Input: part model. Units: mm. Frame: model coordinates. A direction names the side the tool comes from. Coordinates: 2 decimals unless noted, no trailing zeros. Loops run counter-clockwise (first coordinate to the right, second up) from the corner with the lowest first, then second, coordinate; pieces in that order, holes last.
Autodesk Inventor part; units mm, degrees
ref_plane "YZ Plane" through (0, 0, 0) normal (1, 0, 0) x (0, 1, 0)
ref_plane "XZ Plane" through (0, 0, 0) normal (0, 1, 0) x (-1, 0, 0)
ref_plane "XY Plane" through (0, 0, 0) normal (0, 0, 1) x (1, 0, 0)
sketch "Sketch1" plane through (0, 0, 0) normal (0, 0, 1) x (1, 0, 0)
  circle A0 centre (0, 0) radius 8.35 construction
  arc A1 (-8.8064, -7.1064) -> (-5.4064, -7.1064) centre (-7.1064, -7.1064) ccw
  circle A2 centre (7.1064, -7.1064) radius 1.7 construction
  line L0 (0, 12.3642) -> (0, -15.7353)
  line L1 (-7.1064, -8.8064) -> (7.1064, -8.8064) construction
  line L2 (0, 0) -> (7.1064, -7.1064) construction
  line L3 (11.8064, -3.7064) -> (11.8064, -11.7564)
  line L4 (11.8064, -11.7564) -> (-11.8064, -11.7564)
  line L5 (-11.8064, -11.7564) -> (-11.8064, -3.7064)
  circle A3 centre (-7.1064, -3.7064) radius 1.7 construction
  line L6 (-8.8064, -7.1064) -> (-8.8064, -3.7064)
  line L7 (-5.4064, -7.1064) -> (-5.4064, -3.7064)
  line L8 (-11.8064, -3.7064) -> (-8.8064, -3.7064)
  arc A4 (5.4064, -7.1064) -> (8.8064, -7.1064) centre (7.1064, -7.1064) ccw
  line L9 (8.8064, -7.1064) -> (8.8064, -3.7064)
  line L10 (5.4064, -7.1064) -> (5.4064, -3.7064)
  line L11 (-5.4064, -3.7064) -> (5.4064, -3.7064)
  line L12 (8.8064, -3.7064) -> (11.8064, -3.7064)
  dimension "d0" = 16.7
  dimension "d1" = 3.4
  dimension "d4" = 45
  dimension "d5" = 3
  dimension "d6" = 4.65
  dimension "d25" = 17.6129
extrude "Extrusion1" add sketch "Sketch1" along normal blind 60
sketch "Sketch2" plane through (5.4064, -7.1064, 0) normal (1, 0, 0) x (0, 0, -1)
  line L0 (0, -4.65) -> (0, 3.4)
  line L1 (0, 3.4) -> (-60, 3.4)
  line L2 (-60, -4.65) -> (-60, 3.4)
  line L3 (0, -4.65) -> (-60, -4.65)
  line L4 (0, 3.4) -> (-60, 3.4)
  circle A0 centre (-10, 3.4) radius 1.7
  point P0 (0, 7.1064)
  dimension "d9" = 10
  dimension "d10" = 3.4
extrude "Extrusion2" cut sketch "Sketch2" against normal up to surface (10.8128 mm away) contours A0 L1 | L1 A0
pattern_linear "Rectangular Pattern1" count 5 spacing 10 along (0, 0, 1) of "Extrusion2"
sketch "Sketch3" plane through (0, 0, 0) normal (0, 0, -1) x (-1, 0, 0)
  line L0 (11.8064, -3.7064) -> (11.8064, -11.7564)
  line L1 (8.8064, -3.7064) -> (11.8064, -3.7064)
  line L2 (8.8064, -7.1064) -> (8.8064, -3.7064)
  arc A0 (5.4064, -7.1064) -> (8.8064, -7.1064) centre (7.1064, -7.1064) ccw
  line L3 (5.4064, -3.7064) -> (5.4064, -7.1064)
  line L4 (-5.4064, -3.7064) -> (5.4064, -3.7064)
  line L5 (-5.4064, -7.1064) -> (-5.4064, -3.7064)
  arc A1 (-8.8064, -7.1064) -> (-5.4064, -7.1064) centre (-7.1064, -7.1064) ccw
  line L6 (-8.8064, -3.7064) -> (-8.8064, -7.1064)
  line L7 (-11.8064, -3.7064) -> (-8.8064, -3.7064)
  line L8 (-11.8064, -11.7564) -> (-11.8064, -3.7064)
  line L9 (11.8064, -11.7564) -> (-11.8064, -11.7564)
  arc A2 (0.375, -11.4658) -> (-0.375, -11.4658) centre (0, -9.7564) ccw
  line L10 (-0.375, -11.4658) -> (-0.375, -11.7564)
  line L11 (0.375, -11.4658) -> (0.375, -11.7564)
  point P0 (0, 0)
  dimension "d16" = 3.5
  dimension "d17" = 0.75
  dimension "d20" = 2
extrude "Extrusion3" cut sketch "Sketch3" against normal blind 30 contours L9 L10 A2 L11
sketch "Sketch4" plane through (-11.8064, -11.7564, 60) normal (0, -1, 0) x (1, 0, 0)
  line L0 (12.1814, -30) -> (12.1814, -60)
  line L1 (12.1814, -60) -> (23.6128, -60)
  line L2 (23.6128, -60) -> (23.6128, 0)
  line L3 (0, 0) -> (23.6128, 0)
  line L4 (0, -60) -> (0, 0)
  line L5 (0, -60) -> (11.4314, -60)
  line L6 (11.4314, -60) -> (11.4314, -30)
  line L7 (11.4314, -30) -> (12.1814, -30)
  line L8 (13.5064, -30) -> (10.1064, -30)
  line L9 (10.1064, -30) -> (10.1064, -33)
  line L10 (10.1064, -33) -> (13.5064, -33)
  line L11 (13.5064, -33) -> (13.5064, -30)
  line L12 (11.8064, 12) -> (11.8064, -72)
  point P0 (11.8064, -60)
  dimension "d21" = 3.4
  dimension "d22" = 3
extrude "Extrusion4" cut sketch "Sketch4" against normal blind 2 contours L8 L11 L10 L0 | L0 L10 L12 L7 | L12 L10 L6 L7 | L6 L10 L9 L8
sketch "Sketch5" plane through (0, 0, 0) normal (0, 0, -1) x (-1, 0, 0)
  line L0 (-11.8064, -11.7564) -> (-11.8064, -3.7064)
  circle A0 centre (-11.8064, -7.1064) radius 1.7
  line L1 (-0.375, -11.7564) -> (-11.8064, -11.7564)
  line L2 (-11.8064, -3.7064) -> (-8.8064, -3.7064)
  point P0 (0, 0)
  dimension "d26" = 3.4
  dimension "d28" = 3.4
extrude "Extrusion5" cut sketch "Sketch5" against normal up to surface (60 mm away)
sketch "Sketch6" plane through (11.8064, -11.7564, 60) normal (1, 0, 0) x (0, 0, -1)
  line L0 (60, 0) -> (0, 0)
  line L1 (60, 8.05) -> (0, 8.05)
  line L2 (40.7622, 0) -> (40.0122, 0)
  line L3 (40.0122, 0) -> (40.0122, 8.05)
  line L4 (40.0122, 8.05) -> (40.7622, 8.05)
  line L5 (40.7622, 8.05) -> (40.7622, 0)
  line L6 (60, 0) -> (0, 0) construction
  line L7 (40.3872, 0) -> (40.3872, 8.05) construction
  line L8 (60, 8.05) -> (60, 4.65)
  line L9 (60, 2.95) -> (0, 2.95)
  line L10 (60, 6.35) -> (58, 6.35)
  line L11 (58, 6.35) -> (58, 2.95)
  line L12 (58, 2.95) -> (60, 2.95)
  line L13 (60, 2.95) -> (60, 6.35)
  point P0 (60, 11.7564)
  dimension "d31" = 0.75
  dimension "d32" = 2
  dimension "d33" = 17.6129
extrude "Extrusion6" add sketch "Sketch6" against normal blind 1.7 contours L11 L10 L8 L13 L9
extrude "Extrusion7" cut sketch "Sketch6" against normal blind 1.7 contours L0 L3 L9 L5 | L9 L3 L1 L5
pattern_linear "Rectangular Pattern2" count 5 spacing 17.6128 along (0, 0, 1) of "Extrusion7"
sketch "Sketch7" plane through (-5.4064, -3.7064, 11.7) normal (0, 1, 0) x (1, 0, 0)
  point P0 (5.4064, 11.7)
equation "\"d0\" = marbleSize"
equation "\"d1\" = trackDiameter"
equation "\"d10\" = trackDiameter"
equation "\"d21\" = trackDiameter"
equation "\"d26\" = trackDiameter"
equation "\"d28\" = trackDiameter"
equation "\"d29\" = 0.5 * trackDiameter"
equation "\"d33\" = d25"
equation "\"d34\" = 0.5 * trackDiameter"
equation "\"d36\" = 0.5 * trackDiameter"
equation "\"d40\" = d25"
equation "\"marbleSize\" = 16.7"
equation "\"trackDiameter\" = 3.4"
equation "\"numGroove\" = 5"
properties part number "Track Builder"
Item 1: Section query D-D (z = 10). Output: boundary loops of the cut face in (x, y) (3 decimals), then the cut area to 3 significant figures.
Result:
outline: (-11.806, -11.756) - (-0.375, -11.756) - (-0.375, -11.466) arc R1.75 cw (long way) to (0.375, -11.466) - (0.375, -11.756) - (11.806, -11.756) - (11.806, -8.806) arc R1.7 cw to (11.806, -5.406) - (11.806, -3.706) - (8.806, -3.706) - (8.806, -7.106) arc R1.7 cw to (5.406, -7.106) - (5.406, -5.406) - (-5.406, -5.406) - (-5.406, -7.106) arc R1.7 cw to (-8.806, -7.106) - (-8.806, -3.706) - (-11.806, -3.706) - close
area: 125 mm2
Item 2: Section query A-A (z = 40). Output: boundary loops of the cut face in (x, y), then the cut area to 3 significant figures.
Result:
outline: (-11.81, -11.76) - (11.81, -11.76) - (11.81, -8.81) arc R1.7 cw to (11.81, -5.41) - (11.81, -3.71) - (8.81, -3.71) - (8.81, -7.11) arc R1.7 cw to (5.41, -7.11) - (5.41, -5.41) - (-5.41, -5.41) - (-5.41, -7.11) arc R1.7 cw to (-8.81, -7.11) - (-8.81, -3.71) - (-11.81, -3.71) - close
area: 135 mm2
Item 3: Line query: L1, parallel to X at y = -5, z = 12; L2, parallel to X at y = -8.5, z = 49.5; L3, parallel to X at y = -8.5, z = 19. Output: solid intervals per line, ascending.
Result:
L1: x = -11.81 to -8.81, -5.41 to 5.41, 8.81 to 11.81
L2: x = -11.81 to -8.08, -6.13 to 6.13, 8.08 to 10.83
L3: x = -11.81 to -8.08, -6.13 to -1.22, 1.22 to 6.13, 8.08 to 10.83
Item 4: Contact query for a flat-ended pin moving along its axis: P1, Ø1, axis at x = 4, z = 40.5, coming from the +Y side. Output: stop coordinate, or through.
Result:
P1: stops at y = -5.08
Item 5: Section query C-C (y = -10.75). Output: boundary loops of the cut face in (x, z).
Result:
outline: (-11.81, 0) - (-1.44, 0) - (-1.44, 27) - (-1.7, 27) - (-1.7, 30) - (1.7, 30) - (1.7, 27) - (1.44, 27) - (1.44, 0) - (11.81, 0) - (11.81, 19.24) - (10.11, 19.24) - (10.11, 19.99) - (11.81, 19.99) - (11.81, 36.85) - (10.11, 36.85) - (10.11, 37.6) - (11.81, 37.6) - (11.81, 54.46) - (10.11, 54.46) - (10.11, 55.21) - (11.81, 55.21) - (11.81, 60) - (-11.81, 60) - close
Item 6: Mould query, pull axis Z, two halves, no side actions, for faces 1 (the face through (-0.2, -7.7, 0)), 2 (the face through (0.076, -5.406, 30.037)), 3 (the face through (-5.406, -6, 30)), 4 (the face through (0.076, -5.406, 10.037)). Classes: +Z half, -Z half, draft (parallel to the pull), parting line (faces both ways), or undercut.
Result:
face 1: -Z half
face 2: undercut
face 3: draft
face 4: undercut
Item 7: Reachability of faces 5 (the face through (11.806, -9, 10)), 6 (the face through (8.806, -5, 30)), 7 (the face through (0.076, -5.406, 50.037)), 8 (the face through (11, -5, 55.213)), 9 (the face through (10.107, -7.144, 10.498)) from +Z, -Z, +X, -X, +Y, -Y: full face, straight path, thin tool, end or side. Return the list, or none.
Result:
face 5: +Z, -Z, +X, +Y, -Y
face 6: +Z, -Z, +Y
face 7: +Y
face 8: +X, +Y, -Y
face 9: +Z, +X
Item 8: Section query B-B (x = -1). Output: boundary loops of the cut face in (y, z).
Result:
outline: (-11.76, 0) - (-11.19, 0) - (-11.19, 27) - (-11.76, 27) - close; (-11.76, 30) - (-8.32, 30) - (-8.32, 0) - (-3.71, 0) - (-3.71, 8.3) arc R1.7 cw to (-3.71, 11.7) - (-3.71, 18.3) arc R1.7 cw to (-3.71, 21.7) - (-3.71, 28.3) arc R1.7 cw to (-3.71, 31.7) - (-3.71, 38.3) arc R1.7 cw to (-3.71, 41.7) - (-3.71, 48.3) arc R1.7 cw to (-3.71, 51.7) - (-3.71, 60) - (-11.76, 60) - close
